Answer from the drawing. Dimensions are ordinates in mm from the lowest x, y and z of the part. A direction names the side the tool comes from. Coordinates: 2 decimals unless noted, no trailing zeros. Order: outer loops, then holes, each group sorted by start corner. A loop starts at its lowest first (then second) coordinate and runs counter-clockwise, first axis right, second up.
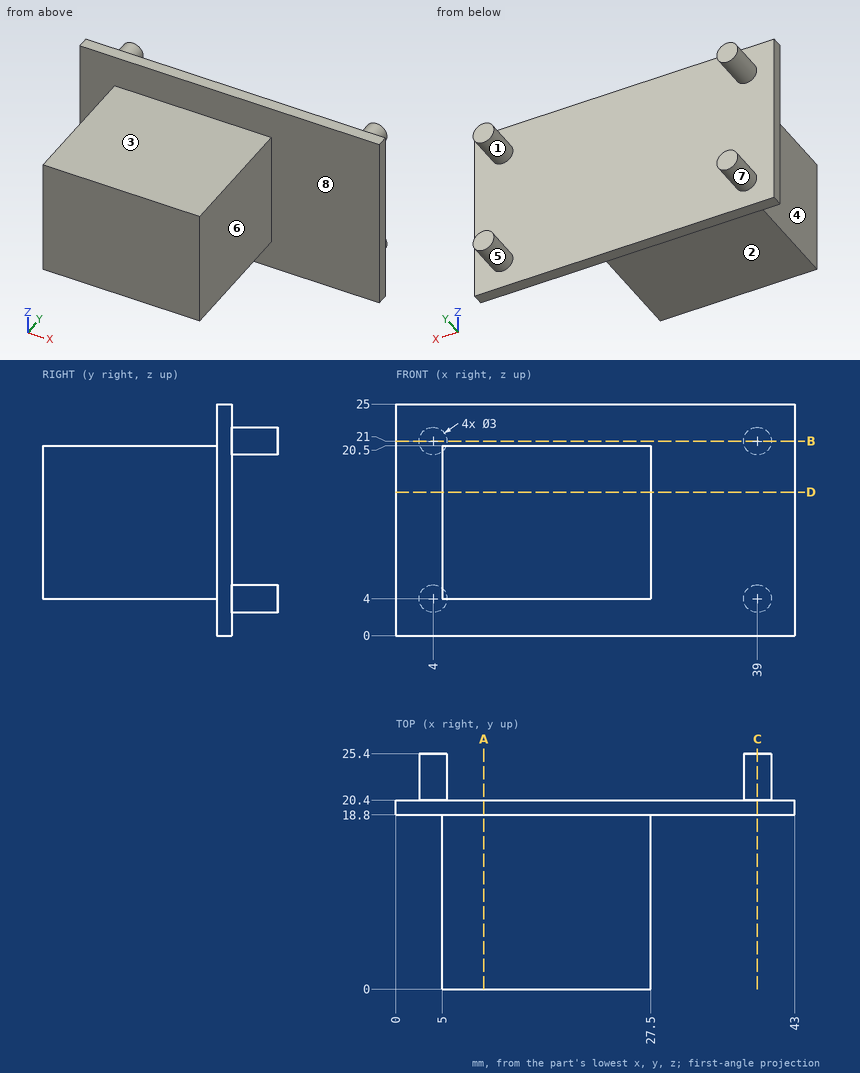
1. For the marked faces 1, 2, 3 and 4, determine the directions among +Z, -Z, +X, -X, +Y, -Y from which every point of the face is accessible in a straight line to the end or side of a thin tool.
2. The mould has two halves that part along X. Classify the marked faces 5, 6, 7 and 8: released by +X, released by -X, zero draft, split by the parting line, or undercut.
3. The part is cut by section D-D (z = 15.5). Determine the outline of the cut face in (x, y).
4. Flat-ended cylindrical pins translate along their axes: pin 1 (8 mm diameter, centred on y = 13.5, z = 10.5, fed in from -X); pin 2 (10 mm diameter, centred on y = 12.5, z = 9.5, fed in from +X); pin 3 (4 mm diameter, centred on x = 6.5, z = 10.5, fed in from -Y); pin 4 (9.5 mm diameter, centred on x = 18.5, y = 14, fed in from +Z). Find the tip coordinate at first contact, or state that the pin passes through.
5. Consider probe 1 along X at (y, z) = (18.75, 5.75); probe 2 along Z at (x, y) = (18.5, 1); probe 3 along Y at (x, z) = (39, 8.25). Determine where each line is inside the solid, lowest interval first.
6. The part is cut by section A-A (x = 9.5). Determine the outline of the cut face in (y, z).
7. The part is cut by section C-C (x = 39). Determine the outline of the cut face in (y, z).
8. The part is cut by section B-B (z = 21). Determine the outline of the cut face in (x, y).
Worked out:
1. face 1: +Y
1. face 2: -Z, +X, -X, -Y
1. face 3: +Z, +X, -X, -Y
1. face 4: +Z, -Z, -X, -Y
2. face 5: undercut
2. face 6: released by +X
2. face 7: undercut
2. face 8: zero draft
3. outline: (0, 18.8) - (5, 18.8) - (5, 0) - (27.5, 0) - (27.5, 18.8) - (43, 18.8) - (43, 20.4) - (0, 20.4) - close
4. pin 1: stops at x = 5
4. pin 2: stops at x = 27.5
4. pin 3: stops at y = 0
4. pin 4: stops at z = 20.5
5. probe 1: x = 5 to 27.5
5. probe 2: z = 4 to 20.5
5. probe 3: y = 18.8 to 20.4
6. outline: (0, 4) - (18.8, 4) - (18.8, 0) - (20.4, 0) - (20.4, 25) - (18.8, 25) - (18.8, 20.5) - (0, 20.5) - close
7. outline: (18.8, 0) - (20.4, 0) - (20.4, 2.5) - (25.4, 2.5) - (25.4, 5.5) - (20.4, 5.5) - (20.4, 19.5) - (25.4, 19.5) - (25.4, 22.5) - (20.4, 22.5) - (20.4, 25) - (18.8, 25) - close
8. outline: (0, 18.8) - (43, 18.8) - (43, 20.4) - (40.5, 20.4) - (40.5, 25.4) - (37.5, 25.4) - (37.5, 20.4) - (5.5, 20.4) - (5.5, 25.4) - (2.5, 25.4) - (2.5, 20.4) - (0, 20.4) - close
